Verification items for the finished model (mm, model axes). Face numbers are marked on the shaded views. A direction names the side the tool comes from. Give positions to 0.01 mm unless a question says otherwise; leave off trailing zeros. Loops run counter-clockwise (first coordinate to the right, second up) from the corner with the lowest first, then second, coordinate; pieces in that order, holes last. Notation, with made-up numbers: (0.25, -20) - (5.25, -20) arc R22 cw to (5.25, 12) - close; hole circle Ø9 at (51, -15). An arc over 180 degrees is marked (long way). Use one line per item in the form item = value.
```python
from build123d import *

# Parameters (mm, degrees)
SKETCH2_W           = 32.2
SKETCH2_H           = 14.5
BOSS_EXTRUDE1_DEPTH = 3
SKETCH3_W           = 19.7
SKETCH3_H           = 2
CUT_EXTRUDE1_DEPTH  = 2.5
SKETCH4_W           = 23.2
SKETCH4_H           = 9
CUT_EXTRUDE2_DEPTH  = 19.648659469
SKETCH5_R           = 1
CUT_EXTRUDE3_DEPTH  = 19.648659469
FILLET1_R           = 1


with BuildPart() as part:
    # Sketch2 → Boss-Extrude1 (new, symmetric)
    with BuildSketch(Plane.XY):
        Rectangle(SKETCH2_W, SKETCH2_H)
    extrude(amount=BOSS_EXTRUDE1_DEPTH, both=True)

    # Sketch3 → Cut-Extrude1 (cut)
    with BuildSketch(Plane(origin=(0, 7.25, 0), x_dir=(1, 0, 0), z_dir=(0, 1, 0))):
        with Locations((-2.25, 0)):
            Rectangle(SKETCH3_W, SKETCH3_H)
    extrude(amount=-CUT_EXTRUDE1_DEPTH, mode=Mode.SUBTRACT)

    # Sketch4 → Cut-Extrude2 (cut, through all)
    with BuildSketch(Plane.XY.offset(3)):
        with Locations((0, -2.75)):
            Rectangle(SKETCH4_W, SKETCH4_H)
    extrude(amount=-CUT_EXTRUDE2_DEPTH, mode=Mode.SUBTRACT)

    # Sketch5 → Cut-Extrude3 (cut, through all)
    with BuildSketch(Plane.XY.offset(3)):
        with Locations((-13.85, -4.25)):
            Circle(SKETCH5_R)
        with Locations((13.85, -4.25)):
            Circle(SKETCH5_R)
    extrude(amount=-CUT_EXTRUDE3_DEPTH, mode=Mode.SUBTRACT)

    # Fillet1
    fillet1_edges = [part.edges().sort_by_distance(p)[0] for p in [
        (-11.6, -7.25, 0),
        (-11.6, 1.75, 0),
        (11.6, 1.75, 0),
        (11.6, -7.25, 0),
        (16.1, -7.25, 0),
        (-16.1, -7.25, 0),
        (-16.1, 7.25, 0),
        (16.1, 7.25, 0),
    ]]
    fillet(fillet1_edges, radius=FILLET1_R)


solid = part.part
```
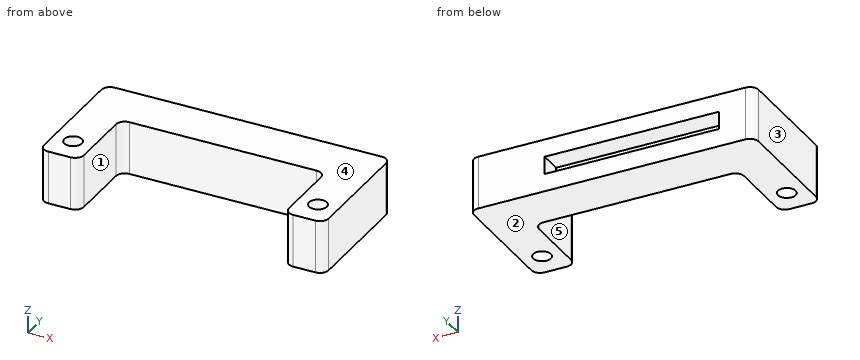
1. Tool access check on the marked faces 1 and 2. Record the directions out of +Z, -Z, +X, -X, +Y, -Y that give a thin tool (end or side, any length) a straight path to the whole face; none if there is none.
Result set:
face_1 = +Z, -Z, -Y
face_2 = -Z, +X, -X, +Y, -Y
2. Scan lines: probe 1 along Y at (x, z) = (13.85, 0.3); probe 2 along X at (y, z) = (-2.25, 0.6); probe 3 along Z at (x, y) = (3.5, 5.25). Record each from-to range of solid material in increasing order.
Result set:
probe_1 = -7.25 to -5.25, -3.25 to 7.25
probe_2 = -16.1 to -11.6, 11.6 to 16.1
probe_3 = -3 to -1, 1 to 3
3. Section check C-C, the plane x = -13.85. Record the cut outline in (y, z).
Result set:
outline = (-7.25, -3) - (-5.25, -3) - (-5.25, 3) - (-7.25, 3) - close; (-3.25, -3) - (7.25, -3) - (7.25, 3) - (-3.25, 3) - close
4. Section check D-D, the plane y = -4.25. Record the cut outline in (x, z).
Result set:
outline = (-16.1, -3) - (-14.85, -3) - (-14.85, 3) - (-16.1, 3) - close; (-12.85, -3) - (-11.6, -3) - (-11.6, 3) - (-12.85, 3) - close; (11.6, -3) - (12.85, -3) - (12.85, 3) - (11.6, 3) - close; (14.85, -3) - (16.1, -3) - (16.1, 3) - (14.85, 3) - close
5. Section check A-A, the plane y = 5.75. Record the cut outline in (x, z), then the cut area to 3 significant figures.
Result set:
outline = (-16.1, -3) - (16.1, -3) - (16.1, 3) - (-16.1, 3) - close; hole (-12.1, -1) - (7.6, -1) - (7.6, 1) - (-12.1, 1) - close
area = 154 mm²
6. Depth check by flat-ended pin: pin 1 Ø2.5 at (x, y) = (13.85, -4.25) entering from +Z; pin 2 Ø2 at (x, z) = (6.5, -2.5) entering from -Y; pin 3 Ø1.2 at (x, y) = (-13.85, -4.25) entering from +Z; pin 4 Ø1 at (x, z) = (-3, 0) entering from +Y. Enter the tip coordinate at first touch or a pass-through.
Result set:
pin_1 = 3
pin_2 = 1.75
pin_3 = through
pin_4 = 4.75
7. Section check B-B, the plane z = 0.5. Record the cut outline in (x, y).
Result set:
outline = (-16.1, -6.25) arc R1 ccw to (-15.1, -7.25) - (-12.6, -7.25) arc R1 ccw to (-11.6, -6.25) - (-11.6, 0.75) arc R1 cw to (-10.6, 1.75) - (10.6, 1.75) arc R1 cw to (11.6, 0.75) - (11.6, -6.25) arc R1 ccw to (12.6, -7.25) - (15.1, -7.25) arc R1 ccw to (16.1, -6.25) - (16.1, 6.25) arc R1 ccw to (15.1, 7.25) - (7.6, 7.25) - (7.6, 4.75) - (-12.1, 4.75) - (-12.1, 7.25) - (-15.1, 7.25) arc R1 ccw to (-16.1, 6.25) - close; hole circle Ø2 at (-13.85, -4.25); hole circle Ø2 at (13.85, -4.25)
8. Draft check along X on the marked faces 3, 4 and 5. Enter one of: released by +X, released by -X, zero draft, split by the parting line, or undercut.
Result set:
face_3 = released by -X
face_4 = zero draft
face_5 = undercut
